```python
from build123d import *

# Parameters (mm, degrees)
PAD010_DEPTH    = 148
SKETCH016_W     = 66.569612
SKETCH016_H     = 138
POCKET005_DEPTH = 33.501
POCKET006_DEPTH = 33.501


with BuildPart() as part:
    # Sketch015 → Pad010 (new body)
    with BuildSketch(Plane.YZ):
        Polygon((-71.9393102292, 47), (-63.2790561914, 42), (-36.1435935394, 89), (-44.8038475773, 94), align=None)
    extrude(amount=PAD010_DEPTH)

    # Sketch016 (on Face2 of Pad010) → Pocket005 (cut, through all)
    with BuildSketch(Plane(origin=(0, -65.645825623, 37.9006350946), x_dir=(0, 0.5, 0.8660254038), z_dir=(0, 0.8660254038, -0.5))):
        with Locations((35.248905, 69)):
            Rectangle(SKETCH016_W, SKETCH016_H)
    extrude(amount=-POCKET005_DEPTH, mode=Mode.SUBTRACT)

    # Sketch017 (on Face3 of Pocket005) → Pocket006 (cut, through all)
    with BuildSketch(Plane(origin=(0, -65.645825623, 37.9006350946), x_dir=(0, 0.5, 0.8660254038), z_dir=(0, 0.8660254038, -0.5))):
        Polygon((4.7335388633, 138), (4.7335388633, 148), (59.0044641671, 148), (59.0044641671, 138), (47.8690015152, 138), (47.8690015152, 141), (15.8690015152, 141), (15.8690015152, 138), align=None)
    extrude(amount=-POCKET006_DEPTH, mode=Mode.SUBTRACT)


solid = part.part
```
Could you check a few things on this model? Use its own coordinates, in mm. Coordinates: 2 decimals unless noted, no trailing zeros. Order: outer loops, then holes, each group sorted by start corner. A loop starts at its lowest first (then second) coordinate and runs counter-clockwise, first axis right, second up. Notation, with made-up numbers: M 89.5,56.25 L 116.5,56.25 A21 cw 116.5,93.25 Z; hole C -3.5,-22 d7. An arc over 180 degrees is marked long. Use one line per item in the form item = value. Start each with the question number.
1. Suppose I cut it at A-A on x = 139.65. Write out the boundary of the cut face in (y, z), then the cut area to 3 significant figures.
2. Please list where these lines run through material, in increasing order: line 1 (Y direction, x = 140.4, z = 75); line 2 (Y direction, x = 140.7, z = 78.5); line 3 (Z direction, x = 140.85, y = -48.75).
3. For pin 1 (10 mm diameter, centred on y = -44.5, z = 73.5, fed in from +X), with a flat end and sliding along its axis, tell me the tip position at first contact or that it passes through.
4. Suppose I cut it at B-B on z = 67. Write out the boundary of the cut face in (x, y).
Geometry says:
q1.outline = M -66.37,56.64 L -57.71,51.64 L -41.71,79.36 L -50.37,84.36 Z
q1.area = 320 mm^2
q2.line_1 = -55.77 to -44.23
q2.line_2 = -53.75 to -42.21
q2.line_3 = 67.17 to 83.42
q3.pin_1 = 141
q4.outline = M 138,-60.39 L 141,-60.39 L 141,-48.85 L 138,-48.85 Z
